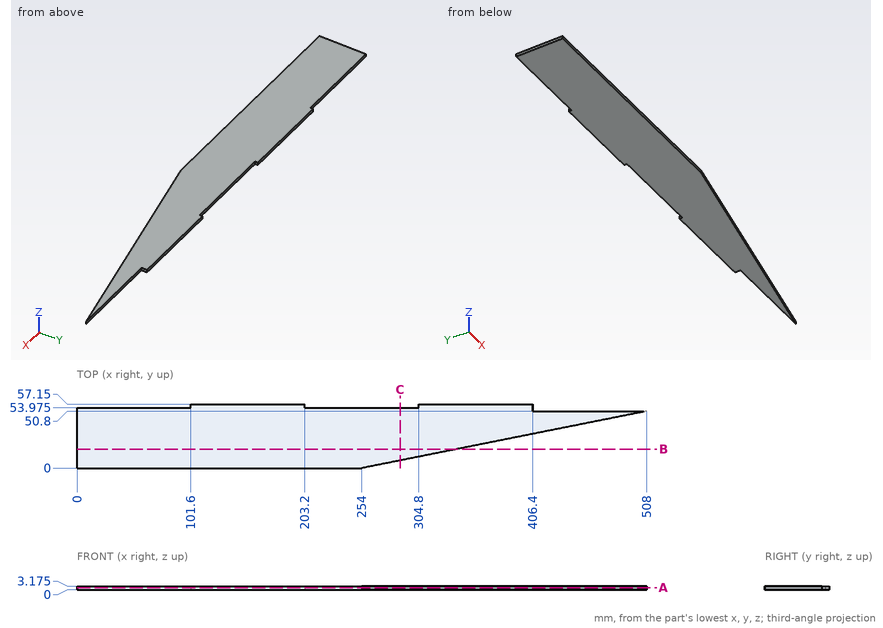
Geometry check sheet. Reference: drawing and pictorial views, mm from the part's lowest x, y, z. Give positions to 0.01 mm unless a question says otherwise; leave off trailing zeros. Order: outer loops, then holes, each group sorted by start corner. A loop starts at its lowest first (then second) coordinate and runs counter-clockwise, first axis right, second up. Notation, with made-up numbers: (-29, 57.5) - (5, 57.5) arc R18 cw to (5, 80.5) - close; hole circle Ø7 at (50.25, 27). An arc over 180 degrees is marked (long way). Answer as CSV lines item,"result".
1. Section check B-B (y = 17). Record the boundary of the cut face in (x, z) (3 decimals), then the cut area to 3 significant figures.
Result sheet:
outline,"(0, 0) - (339, 0) - (339, 3.175) - (0, 3.175) - close"
area,"1,080 mm²"
2. Section check A-A (z = 1.8). Record the boundary of the cut face in (x, y) (3 decimals), then the cut area to 3 significant figures.
Result sheet:
outline,"(0, 0) - (254, 0) - (508, 50.8) - (406.4, 50.8) - (406.4, 57.15) - (304.8, 57.15) - (304.8, 53.975) - (203.2, 53.975) - (203.2, 57.15) - (101.6, 57.15) - (101.6, 53.975) - (0, 53.975) - close"
area,"21,300 mm²"
3. Scan lines: probe 1 along Y at (x, z) = (213, 1.9) (3 decimals); probe 2 along X at (y, z) = (53, 1.5); probe 3 along Y at (x, z) = (482, 2.5). Record each from-to range of solid material in increasing order. Write a range as from..to.
Result sheet:
probe 1,"0..53.975"
probe 2,"0..406.4"
probe 3,"45.6..50.8"
4. Go/stop test with flat-tipped pins: P1, Ø1.6, axis at x = 449, z = 2, coming from the +Y side; P2, Ø1.6, axis at y = 56, z = 2, coming from the +X side; P3, Ø1, axis at y = 56, z = 2, coming from the -X side. Record where each tip stops, or that it passes through.
Result sheet:
P1,"y = 50.8"
P2,"x = 406.4"
P3,"x = 101.6"
5. Section check C-C (x = 288). Record the boundary of the cut face in (y, z) (3 decimals), then the cut area to 3 significant figures.
Result sheet:
outline,"(6.8, 0) - (53.975, 0) - (53.975, 3.175) - (6.8, 3.175) - close"
area,"150 mm²"
